Print and shaded views of the part. All mm, measured from the part's lowest x, y and z. Round coordinates to 2 decimals unless told otherwise and drop trailing zeros. Loops run counter-clockwise (first coordinate to the right, second up) from the corner with the lowest first, then second, coordinate; pieces in that order, holes last. Notation, with made-up numbers: (-4, 82.25) -> (41, 82.25) arc R15 cw to (41, 88.25) -> close; hole circle Ø9 at (-26.75, 21). An arc over 180 degrees is marked (long way). Answer as CSV lines item,"result".
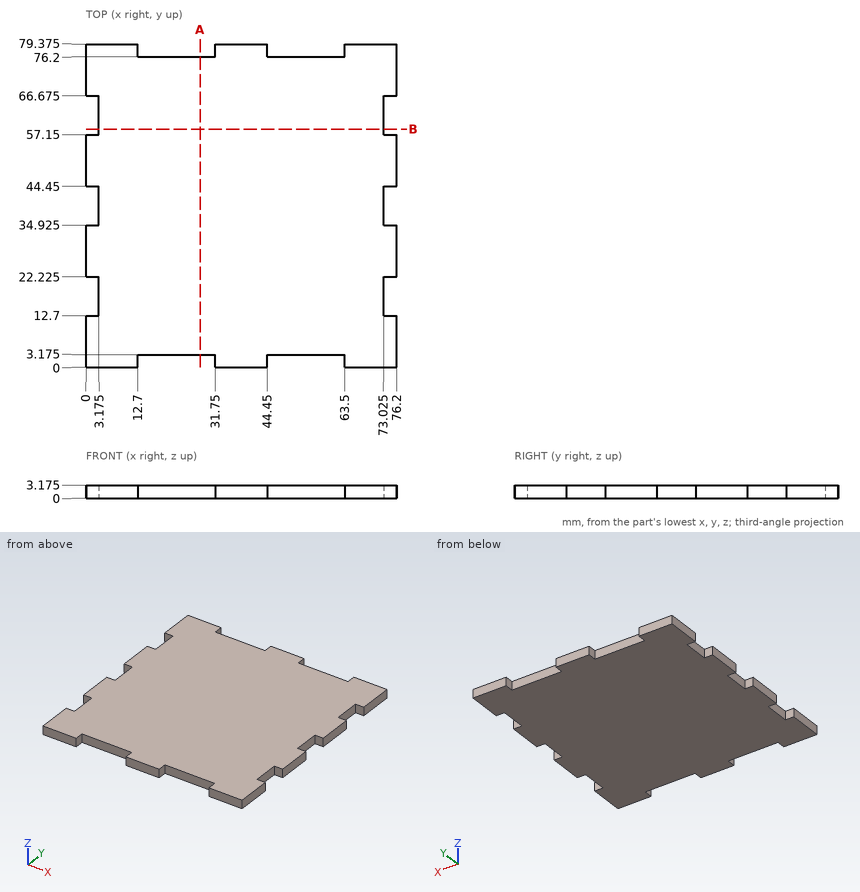
Q1. Slice it at B-B, the plane y = 58.5. Give the cut face in (x, z) (3 decimals).
Results:
outline,"(3.175, 0) -> (73.025, 0) -> (73.025, 3.175) -> (3.175, 3.175) -> close"
Q2. Probe L1, parallel to Y at x = 13, z = 0.7 (3 decimals); L2, parallel to X at y = 43, z = 3 (3 decimals). List the from-to ranges inside material, lowest first. Write a range as [from, to].
Results:
L1,"[3.175, 76.2]"
L2,"[3.175, 73.025]"
Q3. Drop flat-ended pins along their axis: pin 1 Ø1 at (y, z) = (63, 2) entering from +X (3 decimals); pin 2 Ø1.5 at (x, z) = (56.5, 1) entering from +Y; pin 3 Ø1 at (x, z) = (52, 1) entering from -Y (3 decimals). Give the stop position or say it passes through.
Results:
pin 1,"x = 73.025"
pin 2,"y = 76.2"
pin 3,"y = 3.175"
Q4. Slice it at A-A, the plane x = 28. Give the cut face in (y, z) (3 decimals).
Results:
outline,"(3.175, 0) -> (76.2, 0) -> (76.2, 3.175) -> (3.175, 3.175) -> close"
